Geometry check sheet. Reference: drawing and pictorial views, mm from the part's lowest x, y, z. A direction names the side the tool comes from. Round coordinates to 2 decimals unless told otherwise and drop trailing zeros. Loops run counter-clockwise (first coordinate to the right, second up) from the corner with the lowest first, then second, coordinate; pieces in that order, holes last. Notation, with made-up numbers: (18, 68) -> (49, 68) arc R8 ccw to (49, 73) -> close; hole circle Ø10 at (41.5, 48). An arc over 180 degrees is marked (long way). Use one line per item in the form item = value. Start each with the question number.
(1) Set-up check for the marked faces 1, 2 and 3: record each of +Z, -Z, +X, -X, +Y, -Y from which the full face is reachable in a straight line by a thin tool's end or side.
(2) Sectioned sample at B-B (z = 7.5). Record the cut outline in (x, y).
(3) Material ranges on probe 1 along Y at (x, z) = (0.1, 7.5), recorded low to high. Write a range as [from, to].
(4) Go/stop test with flat-tipped pins: pin 1 (0.9 mm diameter, centred on x = 2, z = 7, fed in from -Y); pin 2 (0.9 mm diameter, centred on x = 1, y = 47.5, fed in from +Z); pin 3 (0.9 mm diameter, centred on x = 2, z = 8, fed in from +Y). Record where each tip stops, or that it passes through.
(5) Sectioned sample at A-A (x = 0.85). Record the cut outline in (y, z), and give its area (3 significant figures).
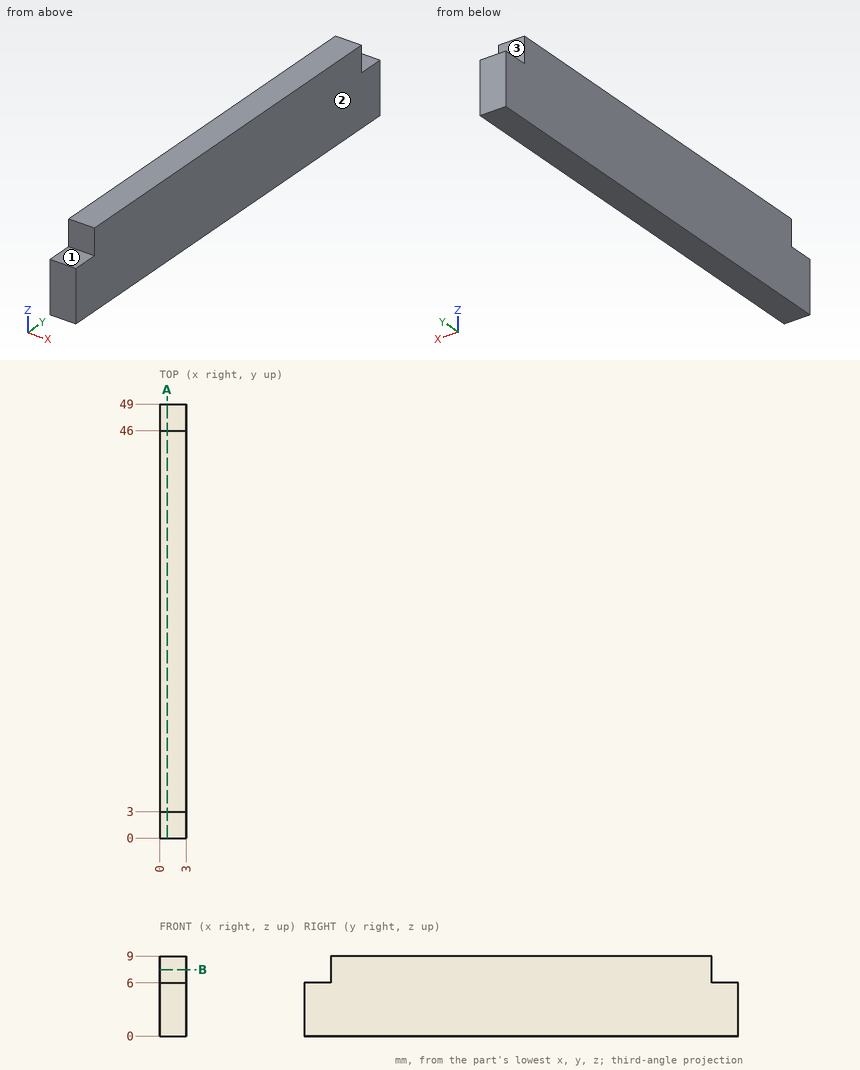
Checks:
q1.face_1 = +Z, +X, -X, -Y
q1.face_2 = +Z, -Z, +X, +Y, -Y
q1.face_3 = +Z, +X, -X, +Y
q2.outline = (0, 3) -> (3, 3) -> (3, 46) -> (0, 46) -> close
q3.probe_1 = [3, 46]
q4.pin_1 = 3
q4.pin_2 = 6
q4.pin_3 = 46
q5.outline = (0, 0) -> (49, 0) -> (49, 6) -> (46, 6) -> (46, 9) -> (3, 9) -> (3, 6) -> (0, 6) -> close
q5.area = 423 mm2
